Could you check a few things on this drawing? It's one solid part, dimensions in mm from its lowest x, y, z. Give positions to 0.01 mm unless a question says otherwise; leave off trailing zeros. Loops run counter-clockwise (first coordinate to the right, second up) from the corner with the lowest first, then second, coordinate; pieces in that order, holes last. Notation, with made-up numbers: M 7.5,46.25 L 18.5,46.25 A31 cw 18.5,70.25 Z; hole C 26.25,12.5 d2. An arc over 180 degrees is marked long. Answer as a JSON object with one key per item and string values.
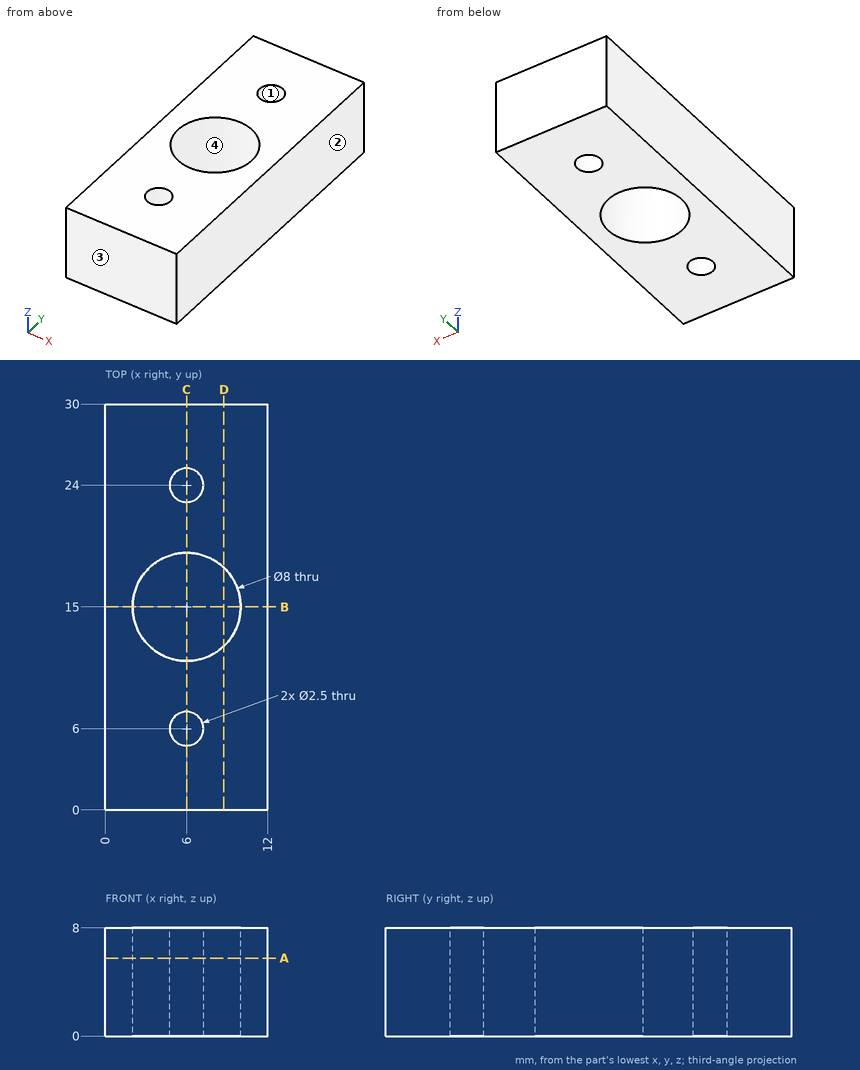
1) Suppose I cut it at C-C, the plane x = 6. Write out the boundary of the cut face in (y, z).
Answer list:
{"outline": "M 0,0 L 4.75,0 L 4.75,8 L 0,8 Z; M 7.25,0 L 11,0 L 11,8 L 7.25,8 Z; M 19,0 L 22.75,0 L 22.75,8 L 19,8 Z; M 25.25,0 L 30,0 L 30,8 L 25.25,8 Z"}
2) Please list where these lines run through material, in increasing order: line 1 along Y through (x, z) = (6, 4.25); line 2 along X through (y, z) = (6, 3.5); line 3 along X through (y, z) = (15, 1.5). Write a range as from..to.
Answer list:
{"line 1": "0..4.75, 7.25..11, 19..22.75, 25.25..30", "line 2": "0..4.75, 7.25..12", "line 3": "0..2, 10..12"}
3) Suppose I cut it at B-B, the plane y = 15. Write out the boundary of the cut face in (x, z), and give its area (3 significant figures).
Answer list:
{"outline": "M 0,0 L 2,0 L 2,8 L 0,8 Z; M 10,0 L 12,0 L 12,8 L 10,8 Z", "area": "32.0 mm^2"}
4) Suppose I cut it at D-D, the plane x = 8.75. Write out the boundary of the cut face in (y, z), and give its area (3 significant figures).
Answer list:
{"outline": "M 0,0 L 12.1,0 L 12.1,8 L 0,8 Z; M 17.9,0 L 30,0 L 30,8 L 17.9,8 Z", "area": "194 mm^2"}
5) If we mould it in two halves opening along Y, with no side actions, what happens to the marked faces 1, 2, 3 and 4? For each: +Y half, -Y half, draft (parallel to the pull), parting line (faces both ways), or undercut.
Answer list:
{"face 1": "undercut", "face 2": "draft", "face 3": "-Y half", "face 4": "undercut"}
6) Suppose I cut it at A-A, the plane z = 5.75. Write out the boundary of the cut face in (x, y).
Answer list:
{"outline": "M 0,0 L 12,0 L 12,30 L 0,30 Z; hole C 6,15 d8; hole C 6,6 d2.5; hole C 6,24 d2.5"}
